from build123d import *

# Parameters (mm, degrees)
SKETCH_1_R          = 6.5
EXTRUDE_1_DEPTH     = 2
SKETCH_2_R          = 3
EXTRUDE_2_DEPTH     = 2
SKETCH_3_R          = 2.25
CUT_EXTRUDE_1_DEPTH = 10
FILLET_2_R          = 0.5
FILLET_3_R          = 0.5


with BuildPart() as part:
    # 草图1 → 凸台-拉伸1 (new body)
    with BuildSketch(Plane(origin=(0, 0, 0), x_dir=(1, 0, 0), z_dir=(0, 1, 0))):
        with Locations(Location((0, 0, 0), (0, 0, 270))):
            Circle(SKETCH_1_R)
    extrude(amount=EXTRUDE_1_DEPTH)

    # 草图2 → 凸台-拉伸2 (add)
    with BuildSketch(Plane(origin=(0, 2, 0), x_dir=(1, 0, 0), z_dir=(0, 1, 0))):
        with Locations(Location((0, 0, 0), (0, 0, 270))):
            Circle(SKETCH_2_R)
    extrude(amount=EXTRUDE_2_DEPTH)

    # 草图3 → 切除-拉伸1 (cut)
    with BuildSketch(Plane(origin=(0, 4, 0), x_dir=(1, 0, 0), z_dir=(0, 1, 0))):
        with Locations(Location((0, 0, 0), (0, 0, 270))):
            Circle(SKETCH_3_R)
    extrude(amount=-CUT_EXTRUDE_1_DEPTH, mode=Mode.SUBTRACT)

    # 圆角2
    fillet_2_edges = [part.edges().sort_by_distance(p)[0] for p in [
        (0, 4, -3),
    ]]
    fillet(fillet_2_edges, radius=FILLET_2_R)

    # 圆角3
    fillet_3_edges = [part.edges().sort_by_distance(p)[0] for p in [
        (0, 2, -6.5),
    ]]
    fillet(fillet_3_edges, radius=FILLET_3_R)


solid = part.part
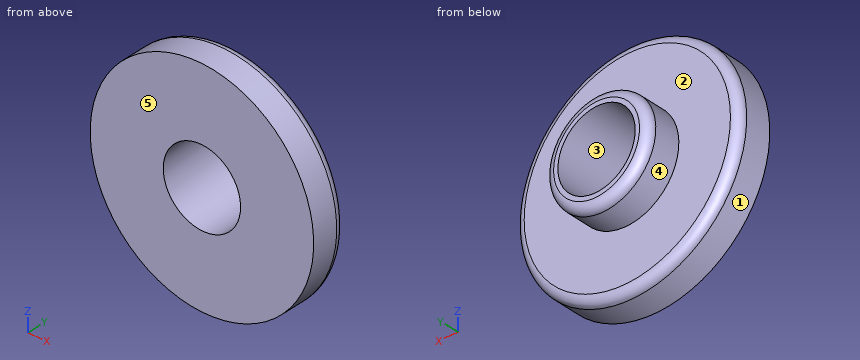
Check sheet for the modelled part. Datum: model origin and axes. Units: mm. Face numbers are marked on the shaded views. A direction names the side the tool comes from. Give positions to 0.01 mm unless a question says otherwise; leave off trailing zeros. Write each loop counter-clockwise with the first axis right and the second up, starting at its lowest first coordinate (ties: lowest second). Pieces come first, ordered by that corner, then holes. Notation, with made-up numbers: (15, 46.25) -> (24, 46.25) arc R14 ccw to (24, 66.25) -> close; hole circle Ø3 at (16, -17). An arc over 180 degrees is marked (long way). One line per item, written item: value. Start each with the question number.
Item 1: Material ranges on probe 1 along X at (y, z) = (2.6, 0); probe 2 along X at (y, z) = (1.55, 0); probe 3 along Y at (x, z) = (4, -4.25), recorded low to high. Write a range as from..to.
Item 2: Section check B-B on z = 0. Record the cut outline in (x, y).
Item 3: Tool access check on the marked faces 4 and 5. Record the directions out of +Z, -Z, +X, -X, +Y, -Y that give a thin tool (end or side, any length) a straight path to the whole face; none if there is none.
Item 4: Section check C-C on y = 3.25. Record the cut outline in (x, z).
Item 5: Section check A-A on x = 0. Record the cut outline in (y, z), then the cut area to 3 significant figures.
Item 6: Draft check along Z on the marked faces 1, 2 and 3. Enter one of: +Z half, -Z half, draft (parallel to the pull), parting line (faces both ways), or undercut.
Item 7: Gauge pin test, flat ends, axial feed: pin 1 (4 mm diameter, centred on x = 4.5, z = 0.5, fed in from -Y); pin 2 (1.5 mm diameter, centred on y = 0.5, z = 1.5, fed in from +X); pin 3 (1.5 mm diameter, centred on x = 3, z = -4.5, fed in from +Y); pin 4 (2 mm diameter, centred on y = 1, z = -2.5, fed in from +X). Record the tip position at first contact, or that the pin passes through.
Results list:
1. probe 1: -3..-2.25, 2.25..3
1. probe 2: -6.5..-2.25, 2.25..6.5
1. probe 3: 0..2
2. outline: (-6.5, 0) -> (-2.25, 0) -> (-2.25, 4) -> (-2.5, 4) arc R0.5 ccw to (-3, 3.5) -> (-3, 2) -> (-6, 2) arc R0.5 ccw to (-6.5, 1.5) -> close; (2.25, 0) -> (6.5, 0) -> (6.5, 1.5) arc R0.5 ccw to (6, 2) -> (3, 2) -> (3, 3.5) arc R0.5 ccw to (2.5, 4) -> (2.25, 4) -> close
3. face 4: +Y
3. face 5: +Z, -Z, +X, -X, -Y
4. outline: circle Ø6 at (0, 0); hole circle Ø4.5 at (0, 0)
5. outline: (0, -6.5) -> (1.5, -6.5) arc R0.5 ccw to (2, -6) -> (2, -3) -> (3.5, -3) arc R0.5 ccw to (4, -2.5) -> (4, -2.25) -> (0, -2.25) -> close; (0, 2.25) -> (4, 2.25) -> (4, 2.5) arc R0.5 ccw to (3.5, 3) -> (2, 3) -> (2, 6) arc R0.5 ccw to (1.5, 6.5) -> (0, 6.5) -> close
5. area: 19.8 mm²
6. face 1: parting line
6. face 2: draft
6. face 3: undercut
7. pin 1: y = 0
7. pin 2: x = 6.46
7. pin 3: y = 2
7. pin 4: x = 6.32
